For this review, use the dimensioned drawing (mm, ordinates from the lowest corner) and the shaded views. A direction names the side the tool comes from. Coordinates: 2 decimals unless noted, no trailing zeros. Write each loop counter-clockwise with the first axis right and the second up, starting at its lowest first coordinate (ties: lowest second). Pieces come first, ordered by that corner, then holes. Notation, with made-up numbers: (-6.5, -28.75) -> (27.5, -28.75) arc R21 ccw to (27.5, -8.75) -> close; hole circle Ø8 at (4.25, 30.25). An arc over 180 degrees is marked (long way). Put each result on its own line as item: value. Start each with the question number.
Item 1: Consider section A-A on z = 9. Give the boundary of the cut face in (x, y).
Item 2: For the marked faces 1 and 2, list the 3-axis set-ups (+Z, -Z, +X, -X, +Y, -Y) from which the entire face can be reached by the end or side of a thin tool; tool diameter is ignored.
Item 3: To check wall thickness, follow L1, parallel to Z at x = 4.5, y = 0.7 (1 decimal); L2, parallel to X at y = 3.25, z = 9; L3, parallel to X at y = 1.5, z = 4. State the ranges of each line that lie inside material, in increasing order.
Item 4: Insertion check: P1, Ø1.2, axis at x = 8.5, z = 8, coming from the +Y side; P2, Ø1, axis at x = 9, y = 3, coming from the -Z side; P3, Ø1.3, axis at x = 13.6, z = 13.6, coming from the -Y side. Each pin has a flat end and moves straight along its axis. Give the tip position at first contact, or say it passes through.
Item 5: Consider section D-D on z = 15. Give the boundary of the cut face in (x, y).
Item 6: The part is to be moulded in two halves that separate along Z. For the marked faces 3, 4, 5 and 6, say which applies: +Z half, -Z half, draft (parallel to the pull), parting line (faces both ways), or undercut.
Item 7: Consider section C-C on y = 0.4. Give the number of separate pieces and of enclosed holes in the cut face, and give its area (3 significant figures).
Item 8: Consider section B-B on x = 15.5. Give the boundary of the cut face in (y, z) (3 decimals).
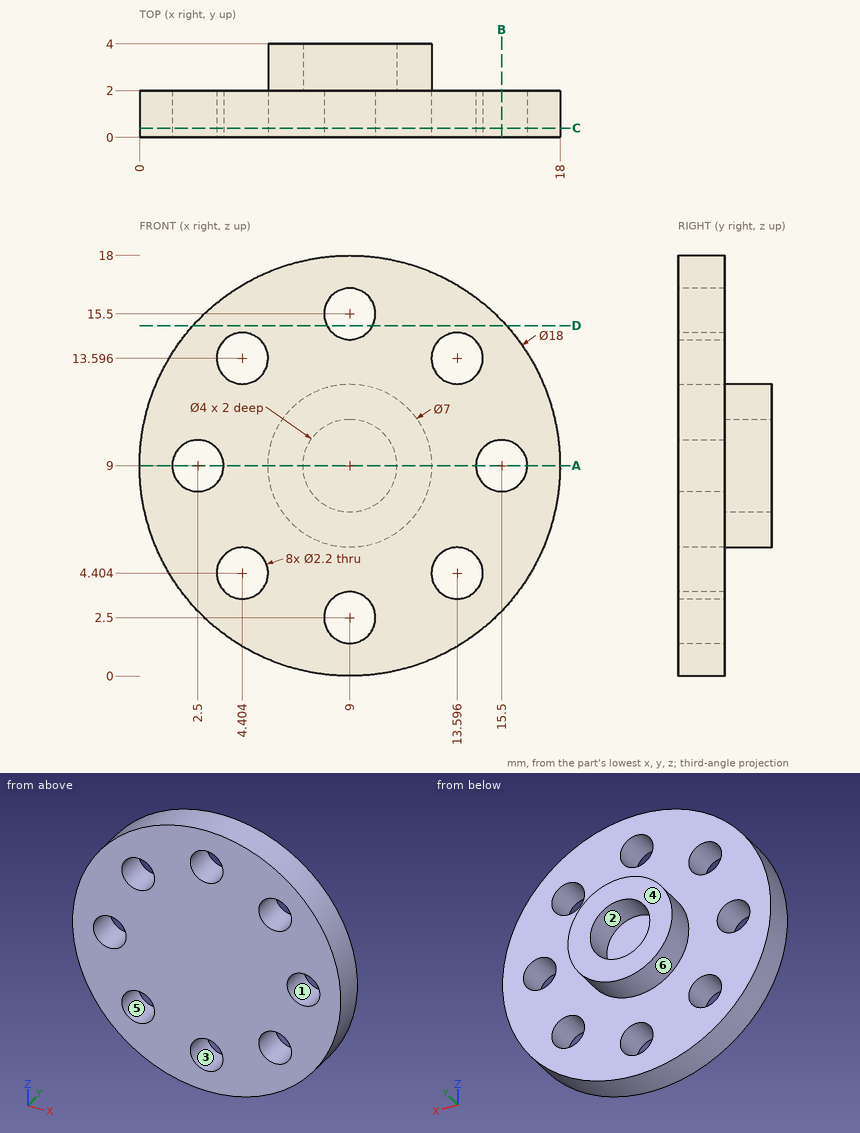
Return value:
1. outline: (0, 0) -> (1.4, 0) -> (1.4, 2) -> (0, 2) -> close; (3.6, 0) -> (14.4, 0) -> (14.4, 2) -> (12.5, 2) -> (12.5, 4) -> (11, 4) -> (11, 2) -> (7, 2) -> (7, 4) -> (5.5, 4) -> (5.5, 2) -> (3.6, 2) -> close; (16.6, 0) -> (18, 0) -> (18, 2) -> (16.6, 2) -> close
2. face 1: +Y, -Y
2. face 2: +Y
3. L1: 1.2 to 3.3, 5.5 to 12.5, 14.7 to 16.8
3. L2: 5.5 to 7, 11 to 12.5
3. L3: 1.52 to 3.38, 5.43 to 12.57, 14.62 to 16.48
4. P1: y = 2
4. P2: z = 5.5
4. P3: through
5. outline: (2.29, 0) -> (8.02, 0) -> (8.02, 2) -> (2.29, 2) -> close; (9.98, 0) -> (15.71, 0) -> (15.71, 2) -> (9.98, 2) -> close
6. face 3: undercut
6. face 4: draft
6. face 5: undercut
6. face 6: parting line
7. separate pieces: 1
7. enclosed holes: 8
7. area: 224 mm^2
8. outline: (0, 2.775) -> (2, 2.775) -> (2, 7.9) -> (0, 7.9) -> close; (0, 10.1) -> (2, 10.1) -> (2, 15.225) -> (0, 15.225) -> close
